```python
from build123d import *

# Parameters (mm, degrees)
PAD004_DEPTH    = 24
SKETCH008_W     = 42
SKETCH008_H     = 1.8
PAD005_DEPTH    = 30
SKETCH010_R     = 2.000122
SKETCH010_R_2   = 2.001214
SKETCH010_R_3   = 2.1
SKETCH010_R_4   = 2.10238
POCKET003_DEPTH = 10


with BuildPart() as part:
    # Sketch006 → Pad004 (new body)
    with BuildSketch(Plane.XZ):
        Polygon((-21.000973, 28), (-29, 28), (-29, -2), (-29, -12), (29, -12), (29, 28), (21, 28), (21, -2), (-21.000973, -2), align=None)
    extrude(amount=PAD004_DEPTH)

    # Sketch008 → Pad005 (join)
    with BuildSketch(Plane(origin=(0, 0, -2), x_dir=(-1, 0, 0), z_dir=(0, 0, 1))):
        with Locations((0, 0.9)):
            Rectangle(SKETCH008_W, SKETCH008_H)
        with Locations((0, 23.1)):
            Rectangle(SKETCH008_W, SKETCH008_H)
    extrude(amount=PAD005_DEPTH)

    # Sketch010 → Pocket003 (cut)
    with BuildSketch(Plane(origin=(0, 0, 28), x_dir=(-1, 0, 0), z_dir=(0, 0, 1))):
        with Locations((-24.9, 17.2)):
            Circle(SKETCH010_R)
        with Locations((-24.9, 7.2)):
            Circle(SKETCH010_R_2)
        with Locations((24.9, 7.2)):
            Circle(SKETCH010_R_3)
        with Locations((25, 17.1)):
            Circle(SKETCH010_R_4)
    extrude(amount=-POCKET003_DEPTH, mode=Mode.SUBTRACT)


solid = part.part
```
The listing builds one solid part. Answer for the finished solid, in the listing's coordinates (mm). A direction names the side the tool comes from. Give positions to 0.01 mm unless a question says otherwise; leave off trailing zeros. Order: outer loops, then holes, each group sorted by start corner. A loop starts at its lowest first (then second) coordinate and runs counter-clockwise, first axis right, second up. Notation, with made-up numbers: (51, 62) -> (59, 62) arc R24 ccw to (59, 99) -> close; hole circle Ø7 at (-32.5, 50). An arc over 180 degrees is marked (long way). One line per item, written item: value.
1) Find section C-C, the plane z = 4.5. Determine the outline of the cut face in (x, y), plus the area to 3 significant figures.
Reported:
outline: (-29, -24) -> (-21, -24) -> (-21, 0) -> (-29, 0) -> close; (-21, -24) -> (29, -24) -> (29, 0) -> (-21, 0) -> (-21, -1.8) -> (21, -1.8) -> (21, -22.2) -> (-21, -22.2) -> close
area: 535 mm^2
2) A flat-ended cylindrical pin translates along its axis: P1, Ø2, axis at x = -25, y = -7.5, coming from the +Z side. Find the tip coordinate at first contact, or state that the pin passes through.
Reported:
P1: stops at z = 18
3) Find section A-A, the plane z = 25. Determine the outline of the cut face in (x, y).
Reported:
outline: (-29, -24) -> (-21, -24) -> (-21, 0) -> (-29, 0) -> close; (-21, -24) -> (29, -24) -> (29, 0) -> (-21, 0) -> (-21, -1.8) -> (21, -1.8) -> (21, -22.2) -> (-21, -22.2) -> close; hole circle Ø4.2 at (-25, -17.1); hole circle Ø4.2 at (-24.9, -7.2); hole circle Ø4 at (24.9, -17.2); hole circle Ø4 at (24.9, -7.2)
4) A tool of negligible diameter and unlimited length cuts with its end or side. For faces 4 (the flat face through (9.9, -1.5, 28)), 5 (the cylindrical face through (26.374, -18.552, 23.07)), from which of +Z, -Z, +X, -X, +Y, -Y can it reach the whole face along a straight path? Write none if from no direction.
Reported:
face 4: +Z, +X, -X, +Y, -Y
face 5: +Z
5) Find section B-B, the plane y = -7.2. Determine the outline of the cut face in (x, z), plus the area to 3 significant figures.
Reported:
outline: (-29, -12) -> (29, -12) -> (29, 28) -> (26.9, 28) -> (26.9, 18) -> (22.9, 18) -> (22.9, 28) -> (21, 28) -> (21, -2) -> (-21, -2) -> (-21, 28) -> (-22.8, 28) -> (-22.8, 18) -> (-27, 18) -> (-27, 28) -> (-29, 28) -> close
area: 978 mm^2
6) Find section D-D, the plane x = 24.9. Determine the outline of the cut face in (y, z), plus the area to 3 significant figures.
Reported:
outline: (-24, -12) -> (0, -12) -> (0, 28) -> (-5.2, 28) -> (-5.2, 18) -> (-9.2, 18) -> (-9.2, 28) -> (-15.2, 28) -> (-15.2, 18) -> (-19.2, 18) -> (-19.2, 28) -> (-24, 28) -> close
area: 880 mm^2
7) Determine the mould class of faces 1 (the flat face through (-21.001, -12, 13)), 2 (the flat face through (0, 0, 8)), 3 (the flat face through (-29, -12, 8)) for opening direction X: pulls with the +X half, pulls with the -X half, needs draft (parallel to the pull), parting line crosses it, or undercut.
Reported:
face 1: undercut
face 2: needs draft
face 3: pulls with the -X half
8) Find the intervals of material crossed by line 1 (Y direction, x = 24.9, z = 22.5); line 2 (X direction, y = -7.2, z = 20.5); line 3 (Y direction, x = 20.5, z = 4.5), in increasing order.
Reported:
line 1: y = -24 to -19.2, -15.2 to -9.2, -5.2 to 0
line 2: x = -29 to -27, -22.8 to -21, 21 to 22.9, 26.9 to 29
line 3: y = -24 to -22.2, -1.8 to 0
